Source: CAD feature listing. Evaluate the final solid. Frame: model axes, mm. Face numbers are marked on the shaded views. A direction names the side the tool comes from. Give positions to 0.01 mm unless a question says otherwise; leave off trailing zeros. Order: outer loops, then holes, each group sorted by start corner. A loop starts at its lowest first (then second) coordinate and runs counter-clockwise, first axis right, second up. Notation, with made-up numbers: (20.5, 23) -> (78.5, 23) arc R22 cw to (78.5, 49) -> close; hole circle Ø9 at (-27.75, 76). An arc over 180 degrees is marked (long way). Answer in a Markdown table with one row per item.
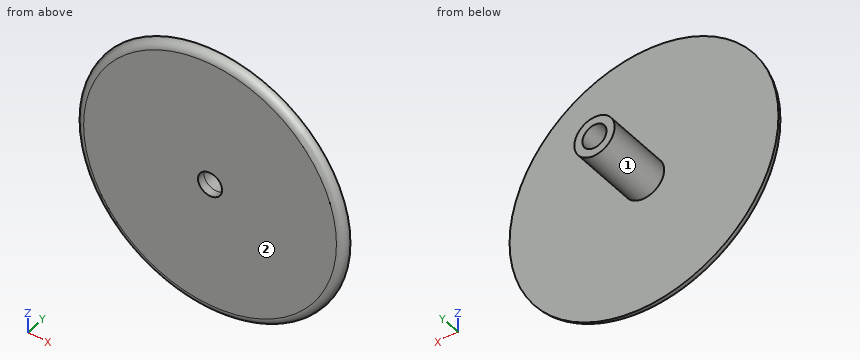
```python
from build123d import *

# Parameters (mm, degrees)
F0_R     = 50.1
F0_R_2   = 4.5
F1_DEPTH = 3
F2_R     = 7.5
F2_R_2   = 4.5
F3_DEPTH = 25
F4_R     = 2.99999


# Not quite as in the source:
# - a fillet or chamfer is up to 0.001 mm smaller than in the source, because OpenCascade refuses the exact size


with BuildPart() as f1:
    # F0 (on Front) → F1 (new body)
    with BuildSketch(Plane.XZ):
        Circle(F0_R)
        Circle(F0_R_2, mode=Mode.SUBTRACT)
    extrude(amount=F1_DEPTH)

    # F2 (on face) → F3 (join)
    with BuildSketch(Plane(origin=(0, 0, 0), x_dir=(-1, 0, 0), z_dir=(0, 1, 0))):
        Circle(F2_R)
        Circle(F2_R_2, mode=Mode.SUBTRACT)
    extrude(amount=F3_DEPTH)

    # F4 (radius 3 in the source; OpenCascade refuses exactly that, so slightly less here)
    f4_edges = [f1.edges().sort_by_distance(p)[0] for p in [
        (-50.1, -3, 0),
    ]]
    fillet(f4_edges, radius=F4_R)


solid = f1.part
```
(1) Section query C-C (y = 2.75). Return the cut outline in (x, z), plus the area to 3 significant figures.
A:
| item | result |
|---|---|
| outline | circle Ø15 at (0, 0); hole circle Ø9 at (0, 0) |
| area | 113 mm^2 |
(2) First-contact query: pin 1 Ø8 at (x, z) = (-37.5, 31.5) entering from -Y; pin 2 Ø1.5 at (x, z) = (-8.5, -33.5) entering from +Y; pin 3 Ø6 at (y, z) = (3.5, 6) entering from +X; pin 4 Ø7 at (x, z) = (0, 0) entering from +Y. Flat tips, straight axial feed; report the tip coordinate or a pass-through.
A:
| item | result |
|---|---|
| pin 1 | stops at y = -3 |
| pin 2 | stops at y = 0 |
| pin 3 | stops at x = 6.87 |
| pin 4 | passes through |
(3) Ray query, probe 1 along Z at (x, y) = (6, 18); probe 2 along Z at (x, y) = (0, 13.5); probe 3 along Y at (x, z) = (19, 9). Return the intervals inside material, ascending.
A:
| item | result |
|---|---|
| probe 1 | z = -4.5 to 4.5 |
| probe 2 | z = -7.5 to -4.5, 4.5 to 7.5 |
| probe 3 | y = -3 to 0 |
(4) Access query for the marked faces 1 and 2. Directions: +Z, -Z, +X, -X, +Y, -Y. A direction counts if a zero-diameter tool reaches every point of the face in a straight line with its end or side. Return the directions, or none.
A:
| item | result |
|---|---|
| face 1 | +Y |
| face 2 | +Z, -Z, +X, -X, -Y |
